Read the model definition and answer for the solid it produces. Units are mm, in the model's axes. Coordinates: 2 decimals unless noted, no trailing zeros. Order: outer loops, then holes, each group sorted by start corner. A loop starts at its lowest first (then second) coordinate and runs counter-clockwise, first axis right, second up.
Autodesk Inventor part; units mm, degrees
ref_plane "YZ Plane" through (0, 0, 0) normal (1, 0, 0) x (0, 1, 0)
ref_plane "XZ Plane" through (0, 0, 0) normal (0, 1, 0) x (-1, 0, 0)
ref_plane "XY Plane" through (0, 0, 0) normal (0, 0, 1) x (1, 0, 0)
sketch "Skizze1" plane through (0, 0, 0) normal (0, 1, 0) x (-1, 0, 0)
  line L0 (-5, 0) -> (-5, 0)
  line L1 (-10, 5) -> (-10, 120)
  line L2 (-10, 120) -> (0, 120)
  line L3 (0, 120) -> (0, 5)
  arc A0 (-5, 0) -> (0, 5) centre (-5, 5) ccw
  arc A1 (-10, 5) -> (-5, 0) centre (-5, 5) ccw
  line L4 (-5, 5) -> (-5, 115.113)
  circle A2 centre (-5, 115.113) radius 2.5
  point P0 (0, 0)
  point P1 (-10, 0)
  dimension "d0" = 10
  dimension "d1" = 120
  dimension "d22" = 5
  dimension "d27" = 110.113
  dimension "d28" = 5
extrude "Extrusion1" add sketch "Skizze1" along normal blind 1 contours L1 L2 L3 A0 A1 | A2
extrude "Extrusion3" cut sketch "Skizze1" along normal blind 10 contours A2
hole "Bohrung3" at (5, 0, 5) direction (0, 1, 0) diameter 5 depth 8 tip angle 118
properties part number "Verbindungsstück_Rolle"
Q1. Determine the mould class of faces 1 (the cylindrical face through (4.249, 0.507, 2.615)), 2 (the cylindrical face through (4.9, 0.5, 0)), 3 (the flat face through (5, 0, 61)) for opening direction X: +X half, -X half, draft (parallel to the pull), parting line (faces both ways), or undercut.
Q2. This flat-tipped pin is pushed along its axis until it touches: P1, Ø4, axis at x = 5, z = 115.113, coming from the -Y side. Where does it stop, or does it pass through?
Q3. The part is cut by section A-A, the plane x = 5. Determine the outline of the cut face in (y, z).
Q4. Straight lines are drawn through the part: L1, parallel to Z at x = 5, y = 0.75; L2, parallel to Z at x = 4.5, y = 0.45; L3, parallel to X at y = 0.3, z = 5. For each, find the intervals that lie inside material, in ascending order.
Q5. The part is cut by section B-B, the plane y = 0.65. Determine the outline of the cut face in (x, z), then the cut area to 3 significant figures.
Computed values:
1. face 1: undercut
1. face 2: parting line
1. face 3: draft
2. P1: passes through
3. outline: (0, 0) - (1, 0) - (1, 2.5) - (0, 2.5) - close; (0, 7.5) - (1, 7.5) - (1, 112.61) - (0, 112.61) - close; (0, 117.61) - (1, 117.61) - (1, 120) - (0, 120) - close
4. L1: z = 0 to 2.5, 7.5 to 112.61, 117.61 to 120
4. L2: z = 0.03 to 2.55, 7.45 to 112.66, 117.56 to 120
4. L3: x = 0 to 2.5, 7.5 to 10
5. outline: (0, 5) arc R5 ccw to (10, 5) - (10, 120) - (0, 120) - close; hole circle Ø5 at (5, 5); hole circle Ø5 at (5, 115.11)
5. area: 1,150 mm2
